For this review, take the finished solid that the model builds, in its own axes (mm). Face numbers are marked on the shaded views. A direction names the side the tool comes from. Coordinates: 2 decimals unless noted, no trailing zeros. Write each loop counter-clockwise with the first axis right and the second up, starting at its lowest first coordinate (ties: lowest second). Pieces come first, ordered by that corner, then holes. Notation, with made-up numbers: (-10, 10) - (46, 10) arc R21 cw to (46, 32) - close; hole circle Ø1 at (24, 56.25). An arc over 180 degrees is marked (long way). Write each question's results on one line, items separated by ' | '.
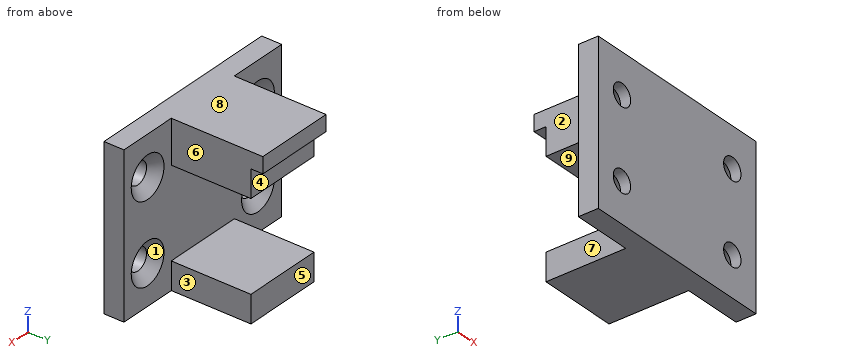
from build123d import *

# Parameters (mm, degrees)
SKETCH1_W                                    = 20
SKETCH1_H                                    = 40
BOSS_EXTRUDE1_DEPTH                          = 25
SKETCH2_W                                    = 20
SKETCH2_H                                    = 4
BOSS_EXTRUDE2_DEPTH                          = 3
SKETCH3_W                                    = 22.23
SKETCH3_H                                    = 20
CUT_EXTRUDE1_DEPTH                           = 20
SKETCH4_W                                    = 15
SKETCH4_H                                    = 40
BOSS_EXTRUDE3_DEPTH                          = 5
CSK_FOR_M5_COUNTERSUNK_FLAT_HEAD_SCR_2_COUNT = 2
CSK_FOR_M5_COUNTERSUNK_FLAT_HEAD_SCR_2_PITCH = 20


with BuildPart() as part:
    # Sketch1 → Boss-Extrude1 (new body)
    with BuildSketch(Plane(origin=(0, 0, 0), x_dir=(1, 0, 0), z_dir=(0, 1, 0))):
        with Locations((10, -20)):
            Rectangle(SKETCH1_W, SKETCH1_H)
    extrude(amount=BOSS_EXTRUDE1_DEPTH)

    # Sketch2 → Boss-Extrude2 (add)
    with BuildSketch(Plane(origin=(0, 25, 0), x_dir=(1, 0, 0), z_dir=(0, 1, 0))):
        with Locations((10, -38)):
            Rectangle(SKETCH2_W, SKETCH2_H)
    extrude(amount=BOSS_EXTRUDE2_DEPTH)

    # Sketch3 → Cut-Extrude1 (cut)
    with BuildSketch(Plane.ZY):
        with Locations((18, 15)):
            Rectangle(SKETCH3_W, SKETCH3_H)
    extrude(amount=-CUT_EXTRUDE1_DEPTH, mode=Mode.SUBTRACT)

    # Sketch4 → Boss-Extrude3 (add)
    with BuildSketch(Plane(origin=(0, 0, 0), x_dir=(1, 0, 0), z_dir=(0, 1, 0))):
        with Locations((-7.5, -20)):
            Rectangle(SKETCH4_W, SKETCH4_H)
    boss_extrude3 = extrude(amount=BOSS_EXTRUDE3_DEPTH)

    # Sketch8 → CSK for M5 Countersunk Flat Head Screw1 (revolve, cut)
    with BuildSketch(Plane(origin=(-7.5, 5, 10), x_dir=(0, 0, 1), z_dir=(1, 0, 0))):
        Polygon((0, 0), (0, 5), (2.75, 5), (2.75, 2.45), (5.2, 0), align=None)
    csk_for_m5_countersunk_flat_head_screw1 = revolve(axis=Axis((-7.5, 11.35, 10), (0, -1, 0)), mode=Mode.SUBTRACT)

    # CSK for M5 Countersunk Flat Head Scr 2: CSK for M5 Countersunk Flat Head Screw1 ×2
    with Locations(*[(0, 0, i * CSK_FOR_M5_COUNTERSUNK_FLAT_HEAD_SCR_2_PITCH) for i in range(1, CSK_FOR_M5_COUNTERSUNK_FLAT_HEAD_SCR_2_COUNT)]):
        add(csk_for_m5_countersunk_flat_head_screw1, mode=Mode.SUBTRACT)

    # Mirror1: Boss-Extrude3, CSK for M5 Countersunk Flat Head Screw1 across plane
    add(boss_extrude3.mirror(Plane.ZY.offset(-10)))
    add(csk_for_m5_countersunk_flat_head_screw1.mirror(Plane.ZY.offset(-10)), mode=Mode.SUBTRACT)

    # Mirror1 copy 1 sketch → Mirror1 copy 1 (revolve, cut)
    with BuildSketch(Plane(origin=(27.5, 5, 30), x_dir=(0, 0, 1), z_dir=(-1, 0, 0))):
        Polygon((0, 0), (0, -5), (2.75, -5), (2.75, -2.45), (5.2, 0), align=None)
    revolve(axis=Axis((27.5, 11.35, 30), (0, 1, 0)), mode=Mode.SUBTRACT)


solid = part.part
Q1. For pin 1 (9 mm diameter, centred on x = 27.5, z = 10, fed in from +Y); pin 2 (5.5 mm diameter, centred on x = 11, z = 5, fed in from +Y); pin 3 (7.5 mm diameter, centred on y = 12.5, z = 4, fed in from +X); pin 4 (3.5 mm diameter, centred on x = -7.5, z = 10, fed in from -Y), all flat-tipped, find the tip position at first contact; note any pin that passes through.
Results found:
pin 1: y = 4.3 | pin 2: y = 25 | pin 3: x = 20 | pin 4: through
Q2. Take a section at A-A on z = 10. State the section outline as (x, y) points, plus the area to 3 significant figures.
Results found:
outline: (-15, 0) - (-10.25, 0) - (-10.25, 2.55) - (-12.7, 5) - (-15, 5) - close; (-4.75, 0) - (24.75, 0) - (24.75, 2.55) - (22.3, 5) - (-2.3, 5) - (-4.75, 2.55) - close; (30.25, 0) - (35, 0) - (35, 5) - (32.7, 5) - (30.25, 2.55) - close | area: 183 mm2
Q3. Take a section at C-C on x = 27.5. State the section outline as (y, z) points.
Results found:
outline: (0, 0) - (5, 0) - (5, 4.8) - (2.55, 7.25) - (0, 7.25) - close; (0, 12.75) - (2.55, 12.75) - (5, 15.2) - (5, 24.8) - (2.55, 27.25) - (0, 27.25) - close; (0, 32.75) - (2.55, 32.75) - (5, 35.2) - (5, 40) - (0, 40) - close
Q4. Take a section at D-D on x = 6. State the section outline as (y, z) points (3 decimals).
Results found:
outline: (0, 0) - (25, 0) - (25, 6.885) - (5, 6.885) - (5, 29.115) - (25, 29.115) - (25, 36) - (28, 36) - (28, 40) - (0, 40) - close
Q5. For the marked faces 5, 6, 7, 8 and 9, list the 3-axis set-ups (+Z, -Z, +X, -X, +Y, -Y) from which the entire face can be reached by the end or side of a thin tool; tool diameter is ignored.
Results found:
face 5: -Z, +X, -X, +Y | face 6: +Z, -Z, +X, +Y | face 7: +Z, -Z, -X, +Y | face 8: +Z, +X, -X, +Y, -Y | face 9: +X, -X, +Y
Q6. Take a section at B-B on y = 11. State the section outline as (x, z) points (3 decimals), plus the area to 3 significant figures.
Results found:
outline: (0, 0) - (20, 0) - (20, 6.885) - (0, 6.885) - close; (0, 29.115) - (20, 29.115) - (20, 40) - (0, 40) - close | area: 355 mm2
Q7. Mouldability with a two-part tool opening along X and no side actions: class the marked faces 1, 2, 3 and 4 as pulls with the +X half, pulls with the -X half, needs draft (parallel to the pull), parting line crosses it, or undercut.
Results found:
face 1: undercut | face 2: pulls with the -X half | face 3: pulls with the +X half | face 4: needs draft
Q8. Wall thickness on line 1 along Z through (x, y) = (-7.5, 1.3); line 2 along X through (y, z) = (0.55, 30); line 3 along Z through (x, y) = (2, 19.5) (3 decimals): over which ranges is each line inside the solid? List them lowest first. Write a range as from..to.
Results found:
line 1: 0..7.25, 12.75..27.25, 32.75..40 | line 2: -15..-10.25, -4.75..24.75, 30.25..35 | line 3: 0..6.885, 29.115..40
